Source: CAD feature listing. Evaluate the final solid. Frame: model axes, mm. Face numbers are marked on the shaded views. A direction names the side the tool comes from. Round coordinates to 2 decimals unless told otherwise and drop trailing zeros. Write each loop counter-clockwise with the first axis right and the second up, starting at its lowest first coordinate (ties: lowest second). Pieces come first, ordered by that corner, then holes.
from build123d import *

# Parameters (mm, degrees)
F0_W     = 60
F0_H     = 60
F1_DEPTH = 71
F2_R     = 2
F3_DEPTH = 10
F4_R     = 4
F5_DEPTH = 24
F7_DEPTH = 16


with BuildPart() as f1:
    # F0 (on Top) → F1 (new body)
    with BuildSketch(Plane.XY):
        Rectangle(F0_W, F0_H)
    extrude(amount=F1_DEPTH)

    # F2 (on face) → F3 (cut)
    with BuildSketch(Plane.XY.offset(71)):
        with Locations((-24.75, -24.75)):
            Circle(F2_R)
        with Locations((24.75, -24.75)):
            Circle(F2_R)
        with Locations((-24.75, 24.75)):
            Circle(F2_R)
        with Locations((24.75, 24.75)):
            Circle(F2_R)
    extrude(amount=-F3_DEPTH, mode=Mode.SUBTRACT)

    # F4 (on face) → F5 (join)
    with BuildSketch(Plane.XY.offset(71)):
        Circle(F4_R)
    extrude(amount=F5_DEPTH)

    # F6 (on face) → F7 (cut)
    with BuildSketch(Plane.XY.offset(95)):
        with BuildLine():
            Line((2.125, 3.3888604279), (4, 0))
            ThreePointArc((4, 0), (3.5, 1.9364916731), (2.125, 3.3888604279))
        make_face()
    extrude(amount=-F7_DEPTH, mode=Mode.SUBTRACT)


solid = f1.part
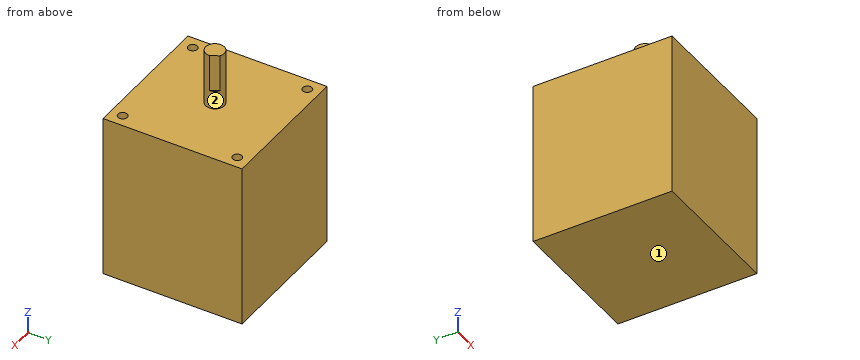
1) Material intervals for line 1 (Y direction, x = 24.75, z = 63.5); line 2 (Y direction, x = -24, z = 67), sorted ascending.
Taken from the geometry:
line 1: y = -30 to -26.75, -22.75 to 22.75, 26.75 to 30
line 2: y = -30 to -26.6, -22.9 to 22.9, 26.6 to 30
2) Section query C-C on y = 20. Return the cut outline in (x, z).
Taken from the geometry:
outline: (-30, 0) - (30, 0) - (30, 71) - (-30, 71) - close
3) Reachability of the marked faces 1 and 2 from +Z, -Z, +X, -X, +Y, -Y: full face, straight path, thin tool, end or side. Return the list, or none.
Taken from the geometry:
face 1: -Z, +X, -X, +Y, -Y
face 2: +Z
4) Section query A-A on y = -24.75. Return the cut outline in (x, z).
Taken from the geometry:
outline: (-30, 0) - (30, 0) - (30, 71) - (26.75, 71) - (26.75, 61) - (22.75, 61) - (22.75, 71) - (-22.75, 71) - (-22.75, 61) - (-26.75, 61) - (-26.75, 71) - (-30, 71) - close
5) Contact query for flat-ended pins moving along their axis: P1, Ø5, axis at x = -24, y = -19, coming from the +Z side; P2, Ø2.5, axis at x = -24.75, y = 24.75, coming from the -Z side; P3, Ø2, axis at y = 4, z = 79.5, coming from the -X side; P4, Ø1.2, axis at x = 24.5, y = 24, coming from the +Z side. Output: stop coordinate, or through.
Taken from the geometry:
P1: stops at z = 71
P2: stops at z = 0
P3: stops at x = -2.65
P4: stops at z = 61
